CAD build for the part. Positions are in the model's coordinates, mm. Coordinates: 2 decimals unless noted, no trailing zeros. Loops run counter-clockwise (first coordinate to the right, second up) from the corner with the lowest first, then second, coordinate; pieces in that order, holes last. Notation, with made-up numbers: (58, 47) - (76, 47) arc R24 ccw to (76, 83) - close; hole circle Ø4 at (49, -11). An arc over 180 degrees is marked (long way). Put each result on its own line as item: value.
```python
from build123d import *

# Parameters (mm, degrees)
SKETCH1_W           = 100
SKETCH1_H           = 100
BOSS_EXTRUDE1_DEPTH = 1.6
SKETCH3_R           = 2.2479
SKETCH3_R_2         = 1.325
SKETCH3_R_3         = 2.25
SKETCH3_R_4         = 2.2
SKETCH3_R_5         = 1.1
CUT_EXTRUDE2_DEPTH  = 2.6
FILLET1_R           = 1
CUT_EXTRUDE4_DEPTH  = 2.6


with BuildPart() as part:
    # Sketch1 → Boss-Extrude1 (new body)
    with BuildSketch(Plane.XY):
        Rectangle(SKETCH1_W, SKETCH1_H)
    extrude(amount=BOSS_EXTRUDE1_DEPTH)

    # Sketch3 → Cut-Extrude2 (cut, through all)
    with BuildSketch(Plane(origin=(0, 0, 1.6), x_dir=(-1, 0, 0), z_dir=(0, 0, -1))):
        Circle(SKETCH3_R)
        with Locations((-34.525, -44.525)):
            Circle(SKETCH3_R_2)
        with Locations((0, -29.25)):
            Circle(SKETCH3_R_3)
        with Locations((-45, -27)):
            Circle(SKETCH3_R_4)
        with Locations((0, 29.25)):
            Circle(SKETCH3_R_3)
        with Locations((-45, 27)):
            Circle(SKETCH3_R_4)
        with Locations((-34.525, 13.525)):
            Circle(SKETCH3_R_2)
        with Locations((15.5, -45.5)):
            Circle(SKETCH3_R_5)
        with Locations((45.5, -45.5)):
            Circle(SKETCH3_R_5)
        with Locations((45.5, -33.5)):
            Circle(SKETCH3_R_5)
        with Locations((-11.475, -44.525)):
            Circle(SKETCH3_R_2)
        with Locations((28.244666378, -9.999429886)):
            Circle(SKETCH3_R_4)
        with Locations((28.244666378, 10.000570114)):
            Circle(SKETCH3_R_4)
    extrude(amount=CUT_EXTRUDE2_DEPTH, mode=Mode.SUBTRACT)

    # Fillet1
    fillet1_edges = [part.edges().sort_by_distance(p)[0] for p in [
        (50, -50, 0.8),
        (-50, -50, 0.8),
        (-50, 50, 0.8),
        (50, 50, 0.8),
    ]]
    fillet(fillet1_edges, radius=FILLET1_R)

    # Sketch5 → Cut-Extrude4 (cut, through all)
    with BuildSketch(Plane(origin=(0, 0, 0), x_dir=(-1, 0, 0), z_dir=(0, 0, -1))):
        Polygon((-14.207463079, 17.79554595), (-17.804907195, 14.265775174), (-18.505268384, 14.979563801), (-14.907824268, 18.509334578), align=None)
    extrude(amount=-CUT_EXTRUDE4_DEPTH, mode=Mode.SUBTRACT)


solid = part.part
```
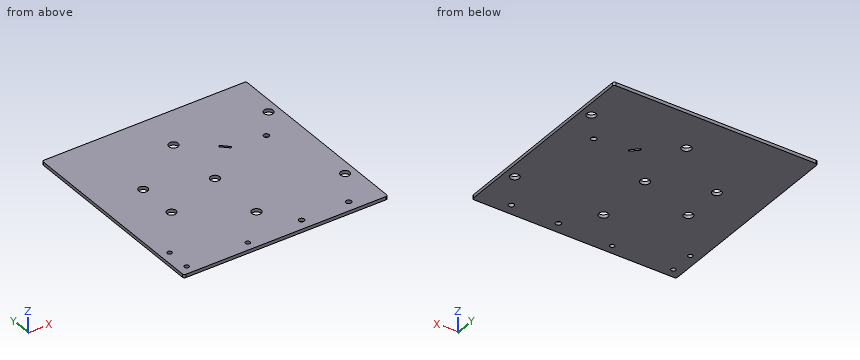
Q1. Slice it at C-C, the plane x = 45. Give the cut face in (y, z), then the cut area to 3 significant figures.
Determined:
outline: (-50, 0) - (-29.2, 0) - (-29.2, 1.6) - (-50, 1.6) - close; (-24.8, 0) - (24.8, 0) - (24.8, 1.6) - (-24.8, 1.6) - close; (29.2, 0) - (50, 0) - (50, 1.6) - (29.2, 1.6) - close
area: 146 mm2
Q2. Slice it at B-B, the plane y = 0. Give the cut face in (x, z), then the cut area to 3 significant figures.
Determined:
outline: (-50, 0) - (-2.25, 0) - (-2.25, 1.6) - (-50, 1.6) - close; (2.25, 0) - (50, 0) - (50, 1.6) - (2.25, 1.6) - close
area: 153 mm2
Q3. Slice it at A-A, the plane x = 0. Give the cut face in (y, z), then the cut area to 3 significant figures.
Determined:
outline: (-50, 0) - (-31.5, 0) - (-31.5, 1.6) - (-50, 1.6) - close; (-27, 0) - (-2.25, 0) - (-2.25, 1.6) - (-27, 1.6) - close; (2.25, 0) - (27, 0) - (27, 1.6) - (2.25, 1.6) - close; (31.5, 0) - (50, 0) - (50, 1.6) - (31.5, 1.6) - close
area: 138 mm2
Q4. Wall check: L1, parallel to Y at x = 0, z = 1.25; L2, parallel to Y at x = -45.5, z = 1.2; L3, parallel to Y at x = -29, z = 0.1. Give the ranges that are in metal, low to high. Write a range as from..to.
Determined:
L1: -50..-31.5, -27..-2.25, 2.25..27, 31.5..50
L2: -50..-46.6, -44.4..-34.6, -32.4..50
L3: -50..-12.07, -7.93..7.93, 12.07..50
